Work out the finished part from the listing and answer in its coordinate system (mm). A direction names the side the tool comes from. Give positions to 0.01 mm unless a question says otherwise; leave off trailing zeros. Loops run counter-clockwise (first coordinate to the right, second up) from the corner with the lowest first, then second, coordinate; pieces in that order, holes last. Notation, with made-up numbers: (27.5, -2.75) -> (77.5, -2.75) arc R10 cw to (77.5, 9.25) -> close; hole circle Ø4 at (69, -37). An arc over 180 degrees is marked (long way). Answer as CSV lines item,"result". Start each with the question number.
1. Find section A-A, the plane x = 0. Give the vertices of the cut face in (y, z) (3 decimals), and give its area (3 significant figures).
2. A tool of negligible diameter and unlimited length cuts with its end or side. For faces 1 (the face through (-1.2, 0, 1.2)), 2 (the face through (0.879, -1.007, -0.517)), 3 (the face through (0, 5, 0)), from which of +Z, -Z, +X, -X, +Y, -Y can it reach the whole face along a straight path? Write none if from no direction.
3. Find the intervals of material crossed by line 1 along Y through (x, z) = (0.1, -0.65); line 2 along X through (y, z) = (2.75, 0); line 3 along Z through (x, y) = (-0.3, -1), in increasing order.
4. Flat-ended cylindrical pins translate along their axes: pin 1 Ø0.8 at (x, y) = (0.5, -1) entering from -Z; pin 2 Ø1 at (y, z) = (1, 0.5) entering from +X. Find the tip coordinate at first contact, or state that the pin passes through.
5. Find section C-C, the plane y = -0.75. Give the vertices of the cut face in (x, z).
6. Find section B-B, the plane z = -1.2. Give the vertices of the cut face in (x, y), and give its area (3 significant figures).
7. Find section D-D, the plane y = 4. Give the vertices of the cut face in (x, z).
8. Determine the mould class of faces 4 (the face through (0.45, 2.46, 1.43)), 5 (the face through (0.89, -1.01, 0.5)), 6 (the face through (-1, -1.5, 1)) for opening direction Z: +Z half, -Z half, draft (parallel to the pull), parting line (faces both ways), or undercut.
from build123d import *

# Parameters (mm, degrees)
SKETCH_1_R          = 1.5
EXTRUDE_1_DEPTH     = 2
SKETCH_2_R          = 2.775
EXTRUDE_2_DEPTH     = 1.5
CUT_EXTRUDE_1_DEPTH = 1
SKETCH_1_8_R        = 1.5
EXTRUDE_5_DEPTH     = 5


with BuildPart() as part:
    # Sketch 1 → Extrude 1 (new body)
    with BuildSketch(Plane(origin=(0, 0, 0), x_dir=(1, 0, 0), z_dir=(0, 1, 0))):
        with Locations(Location((0, 0, 0), (0, 0, 270))):
            Circle(SKETCH_1_R)
    extrude(amount=EXTRUDE_1_DEPTH)

    # Sketch 2 → Extrude 2 (add)
    with BuildSketch(Plane(origin=(0, 0, 0), x_dir=(-1, 0, 0), z_dir=(0, 1, 0))):
        with Locations(Location((0, 0, 0), (0, 0, 90))):
            Circle(SKETCH_2_R)
    extrude(amount=-EXTRUDE_2_DEPTH)

    # Sketch 4 → Cut-Revolve 1 (revolve, cut)
    with BuildSketch(Plane(origin=(0, 0, 0), x_dir=(0, 0, -1), z_dir=(1, 0, 0))):
        with BuildLine():
            Line((-2.775, 0), (-2.775, -1.5))
            Line((-2.775, -1.5), (-2, -1.5))
            ThreePointArc((-2, -1.5), (-2.50252997, -0.809432151), (-2.775, 0))
        make_face()
    revolve(axis=Axis((0, 3.165730861, 0), (0, -1, 0)), mode=Mode.SUBTRACT)

    # Sketch 3 → Cut-Extrude 1 (cut)
    with BuildSketch(Plane.XZ.offset(1.5)):
        Polygon((-1.177794549, 0), (-0.588897275, -1.02), (0.588897275, -1.02), (1.177794549, 0), (0.588897275, 1.02), (-0.588897275, 1.02), align=None)
    extrude(amount=-CUT_EXTRUDE_1_DEPTH, mode=Mode.SUBTRACT)

    # Sketch 1_8 → Extrude 5 (add)
    with BuildSketch(Plane(origin=(0, 0, 0), x_dir=(1, 0, 0), z_dir=(0, 1, 0))):
        with Locations(Location((0, 0, 0), (0, 0, 270))):
            Circle(SKETCH_1_8_R)
    extrude(amount=EXTRUDE_5_DEPTH)


solid = part.part
Resolved:
1,outline,"(-1.5, -2) arc R2.817 ccw to (0, -2.775) -> (0, -1.5) -> (5, -1.5) -> (5, 1.5) -> (0, 1.5) -> (0, 2.775) arc R2.817 ccw to (-1.5, 2) -> (-1.5, 1.02) -> (-0.5, 1.02) -> (-0.5, -1.02) -> (-1.5, -1.02) -> close"
1,area,"20.4 mm^2"
2,face 1,"+Y"
2,face 2,"-Y"
2,face 3,"+Z, -Z, +X, -X, +Y"
3,line 1,"y = -0.5 to 5"
3,line 2,"x = -1.5 to 1.5"
3,line 3,"z = -2.38 to -1.02, 1.02 to 2.38"
4,pin 1,"stops at z = -2.56"
4,pin 2,"stops at x = 1.5"
5,outline,"circle Ø5.06 at (0, 0); hole (-1.18, 0) -> (-0.59, -1.02) -> (0.59, -1.02) -> (1.18, 0) -> (0.59, 1.02) -> (-0.59, 1.02) -> close"
6,outline,"(-2.5, 0) arc R2.55 ccw to (-1.6, -1.5) -> (1.6, -1.5) arc R2.55 ccw to (2.5, 0) -> (0.9, 0) -> (0.9, 5) -> (-0.9, 5) -> (-0.9, 0) -> close"
6,area,"15.5 mm^2"
7,outline,"circle Ø3 at (0, 0)"
8,face 4,"parting line"
8,face 5,"undercut"
8,face 6,"draft"
